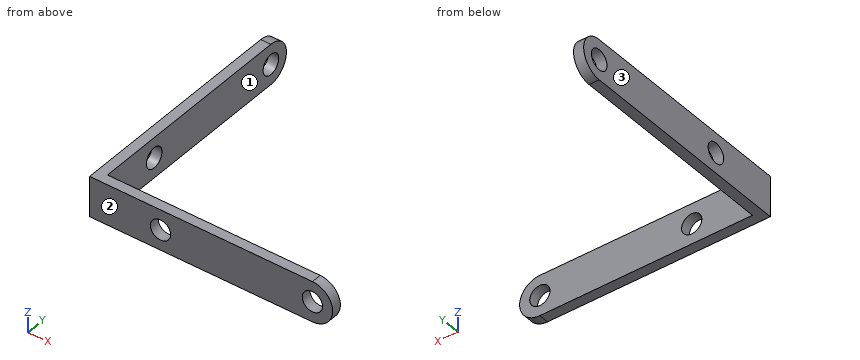
```python
from build123d import *

# Parameters (mm, degrees)
SKETCH115_R            = 1
PAD074_DEPTH           = 1
SKETCH116_R            = 1
PAD075_DEPTH           = 1
FUSION_PLACEMENT_ANGLE = 90


with BuildPart() as flat:
    # Sketch115 → Pad074 (new body)
    with BuildSketch(Plane.XY):
        with BuildLine():
            Line((0, 22), (0, 0))
            Line((0, 0), (4, 0))
            Line((4, 0), (4, 22))
            ThreePointArc((4, 22), (2, 24), (0, 22))
        make_face()
        with Locations((2, 22)):
            Circle(SKETCH115_R, mode=Mode.SUBTRACT)
        with Locations((2, 7)):
            Circle(SKETCH115_R, mode=Mode.SUBTRACT)
    extrude(amount=PAD074_DEPTH)


with BuildPart() as high:
    # Pad075 base: copy of Flat
    add(flat.part)

    # Sketch116 → Pad075 (new body)
    with BuildSketch(Plane.XZ.offset(-1)):
        with BuildLine():
            Line((0, 22), (0, 0))
            Line((0, 0), (4, 0))
            Line((4, 0), (4, 22))
            ThreePointArc((4, 22), (2, 24), (0, 22))
        make_face()
        with Locations((2, 22)):
            Circle(SKETCH116_R, mode=Mode.SUBTRACT)
        with Locations((2, 7)):
            Circle(SKETCH116_R, mode=Mode.SUBTRACT)
    extrude(amount=PAD075_DEPTH)


with BuildPart() as fusion:
    # Fusion base: copy of Flat
    add(flat.part)

    # Fusion: union High
    add(high.part)


with BuildPart() as fusion_1:
    # Fusion placement: moved
    add(fusion.part.moved(Location((2, 0, 52))).rotate(Axis((2, 0, 52), (0, 1, 0)), FUSION_PLACEMENT_ANGLE))


solid = fusion_1.part
```
Input: part model. Units: mm. Frame: model coordinates. Face numbers are marked on the shaded views. Round coordinates to 2 decimals unless told otherwise and drop trailing zeros. Loops run counter-clockwise (first coordinate to the right, second up) from the corner with the lowest first, then second, coordinate; pieces in that order, holes last. Notation, with made-up numbers: (21, 56) - (60, 56) arc R27 cw to (60, 72) - close; hole circle Ø6 at (52.5, -29). An arc over 180 degrees is marked (long way). One line per item, written item: value. Start each with the question number.
(1) Ray query, line 1 (X direction, y = 0.35, z = 50); line 2 (Y direction, x = 2.4, z = 50); line 3 (Y direction, x = 11.5, z = 48.35). Return the intervals inside material, ascending. Write a range as [from, to].
(2) Section D-D, the plane y = 3. Return loops of the section in (x, z), plus the area to 3 significant figures.
(3) Section A-A, the plane y = 7. Return loops of the section in (x, z), plus the area to 3 significant figures.
(4) Section C-C, the plane x = 9. Return loops of the section in (y, z).
(5) Contact query for a flat-ended pin moving along its axis: P1, Ø1, axis at x = 9, z = 51, coming from the +Y side. Output: stop coordinate, or through.
(6) Draft query along X for the marked faces 1, 2 and 3. Return one class per face: +X half, -X half, draft (parallel to the pull), parting line (faces both ways), or undercut.
(7) Section B-B, the plane z = 50. Return loops of the section in (x, y), plus the area to 3 significant figures.
Results below:
1. line 1: [2, 8], [10, 23], [25, 26]
1. line 2: [0, 6], [8, 21], [23, 24]
1. line 3: [0, 1]
2. outline: (2, 48) - (3, 48) - (3, 52) - (2, 52) - close
2. area: 4.00 mm^2
3. outline: (2, 48) - (3, 48) - (3, 49) - (2, 49) - close; (2, 51) - (3, 51) - (3, 52) - (2, 52) - close
3. area: 2.00 mm^2
4. outline: (0, 48) - (1, 48) - (1, 49) - (0, 49) - close; (0, 51) - (1, 51) - (1, 52) - (0, 52) - close
5. P1: y = 1
6. face 1: +X half
6. face 2: draft
6. face 3: -X half
7. outline: (2, 0) - (8, 0) - (8, 1) - (3, 1) - (3, 6) - (2, 6) - close; (2, 8) - (3, 8) - (3, 21) - (2, 21) - close; (2, 23) - (3, 23) - (3, 24) - (2, 24) - close; (10, 0) - (23, 0) - (23, 1) - (10, 1) - close; (25, 0) - (26, 0) - (26, 1) - (25, 1) - close
7. area: 39.0 mm^2
